Autodesk Inventor part; units mm, degrees
ref_plane "YZ Plane" through (0, 0, 0) normal (1, 0, 0) x (0, 1, 0)
ref_plane "XZ Plane" through (0, 0, 0) normal (0, 1, 0) x (-1, 0, 0)
ref_plane "XY Plane" through (0, 0, 0) normal (0, 0, 1) x (1, 0, 0)
sketch "Sketch2" plane through (0, 0, 0) normal (0, 1, 0) x (-1, 0, 0)
  circle A0 centre (0, 0) radius 9
  dimension "d0" = 18
extrude "Extrusion1" add sketch "Sketch2" along normal blind 35
sketch "Sketch3" plane through (0, 0, 0) normal (0, -1, 0) x (1, 0, 0)
  circle A0 centre (0, 0) radius 15
  dimension "d3" = 30
extrude "Extrusion2" add sketch "Sketch3" along normal blind 35
sketch "Sketch4" plane through (0, -35, 0) normal (0, -1, 0) x (1, 0, 0)
  circle A0 centre (0, 0) radius 9
  circle A1 centre (0, 0) radius 9
extrude "Extrusion3" add sketch "Sketch4" along normal blind 5
ref_plane "Work Plane1" through (0, -40, 0) normal (0, 0, -1) x (-1, 0, 0)
sketch "Sketch7" plane through (0, -40, 0) normal (0, 0, -1) x (-1, 0, 0)
  point P0 (0, 40)
sketch "Sketch8" plane through (0, -40, 0) normal (0, 0, -1) x (-1, 0, 0)
  line L0 (-9, 0) -> (9, 0)
  line L1 (-15, 5) -> (15, 5)
  line L2 (0, 0) -> (15, 0) construction
  line L3 (-16.3397, 0) -> (-25, -5)
  line L4 (0, 0) -> (0, -5)
  line L5 (0, -5) -> (-25, -5)
  line L6 (0, 0) -> (-16.3397, 0)
  point P0 (0, 40)
  dimension "d21" = 5
  dimension "d22" = 25
revolve "Revolution1" add sketch "Sketch8" angle 360 about axis through (0, -40, 0) along (0, -1, 0)
sketch "Sketch9" plane through (0, -45, 0) normal (0, -1, 0) x (1, 0, 0)
  circle A0 centre (0, 0) radius 25
extrude "Extrusion5" add sketch "Sketch9" along normal blind 5
sketch "Sketch10" plane through (0, -50, 0) normal (0, -1, 0) x (1, 0, 0)
  circle A0 centre (0, 0) radius 20
  dimension "d26" = 40
extrude "Extrusion6" add sketch "Sketch10" along normal blind 10
sketch "Sketch11" plane through (0, -60, 0) normal (0, -1, 0) x (1, 0, 0)
  circle A0 centre (0, 0) radius 9
  circle A1 centre (0, 0) radius 12
  dimension "d29" = 24
extrude "Extrusion7" add sketch "Sketch11" along normal blind 15 contours A0 | A1
sketch "Sketch12" plane through (0, 35, 0) normal (0, 1, 0) x (1, 0, 0)
  circle A0 centre (0, 0) radius 6
  dimension "d32" = 12
extrude "Extrusion8" cut sketch "Sketch12" against normal blind 120
sketch "Sketch13" plane through (0, -40, 0) normal (0, 0, -1) x (-1, 0, 0)
  circle A0 centre (0, 55) radius 6
  line L0 (9, 75) -> (-9, 75)
  line L1 (9, 40) -> (-9, 40)
  point P0 (0, 40)
  dimension "d45" = 12
  dimension "d47" = 15
extrude "Extrusion9" cut sketch "Sketch13" along normal mid plane 18
move or copy body "Move Body2" bodies to move or copy 1 copy no rotation origin (0, 0, 0) rotation axis (0, 1, 0) rotation angle -90
chamfer "Chamfer1" distance 2 angle 45 1 edges at (0, -75, -12)
properties part number "Vtulka"
Check sheet for the modelled part. Datum: model origin and axes. Units: mm. A direction names the side the tool comes from. Give positions to 0.01 mm unless a question says otherwise; leave off trailing zeros. Order: outer loops, then holes, each group sorted by start corner. A loop starts at its lowest first (then second) coordinate and runs counter-clockwise, first axis right, second up. Notation, with made-up numbers: (54, 20.5) -> (104, 20.5) arc R17 cw to (104, 46.5) -> close; hole circle Ø3 at (14.5, 50). An arc over 180 degrees is marked (long way). Return JSON: item names as keys, results as strings.
1. Cross-section at B-B, the plane y = -18. Record the cut outline in (x, z).
From the geometry:
{"outline": "circle Ø30 at (0, 0); hole circle Ø12 at (0, 0)"}
2. Material ranges on probe 1 along X at (y, z) = (24, 0); probe 2 along X at (y, z) = (-29.5, 0), recorded low to high. Write a range as [from, to].
From the geometry:
{"probe 1": "[-9, -6], [6, 9]", "probe 2": "[-15, -6], [6, 15]"}
3. Cross-section at D-D, the plane y = -47. Record the cut outline in (x, z).
From the geometry:
{"outline": "circle Ø50 at (0, 0); hole circle Ø12 at (0, 0)"}
4. Mould release check, pull along X, two halves, no side actions. Record for faces 4 (the cylindrical face through (-2.3, 27.36, 5.54)), 5 (the flat face through (9, -60, 9)), 6 (the cylindrical face through (7.509, -47.465, 23.846)): +X half, -X half, draft (parallel to the pull), parting line (faces both ways), or undercut.
From the geometry:
{"face 4": "undercut", "face 5": "draft", "face 6": "parting line"}
5. Go/stop test with flat-tipped pins: P1, Ø19, axis at y = 15, z = 0, coming from the -X side; P2, Ø10, axis at x = 15, z = -14, coming from the -Y side; P3, Ø2, axis at x = -17.5, y = -0.5, coming from the +Z side; P4, Ø1.5, axis at y = -14.5, z = 5.5, coming from the +X side. Record where each tip stops, or that it passes through.
From the geometry:
{"P1": "x = -9", "P2": "y = -60", "P3": "through", "P4": "x = 14.23"}
6. Set-up check for faces 1 (the flat face through (6.5, 0, 6.5)), 2 (the flat face through (7, -40, 7)), 3 (the cylindrical face through (-19.524, -54.93, -4.336)): record each of +Z, -Z, +X, -X, +Y, -Y from which the full face is reachable in a straight line by a thin tool's end or side.
From the geometry:
{"face 1": "+Y", "face 2": "none", "face 3": "-Y"}
7. Cross-section at A-A, the plane y = 18.5. Record the cut outline in (x, z).
From the geometry:
{"outline": "(-7.57, -4.87) arc R9 ccw to (7.57, -4.87) -> (3.5, -4.87) arc R6 cw to (-3.5, -4.87) -> close; (-7.57, 4.87) -> (-3.5, 4.87) arc R6 cw to (3.5, 4.87) -> (7.57, 4.87) arc R9 ccw to start"}
8. Cross-section at C-C, the plane z = 0. Count the separate pieces of the cut face and the enclosed holes in it, plus the area to 3 significant figures.
From the geometry:
{"separate pieces": "4", "enclosed holes": "0", "area": "1,590 mm^2"}
